Check sheet for the modelled part. Datum: model origin and axes. Units: mm. Round coordinates to 2 decimals unless told otherwise and drop trailing zeros. Order: outer loops, then holes, each group sorted by start corner. A loop starts at its lowest first (then second) coordinate and runs counter-clockwise, first axis right, second up. Notation, with made-up numbers: (28.25, 29) -> (74.25, 29) arc R17 cw to (74.25, 61) -> close; hole circle Ø3 at (-34, 3.25). An arc over 180 degrees is marked (long way). Use CSV: the item, a comma, the result in double quotes.
```python
from build123d import *

# Parameters (mm, degrees)
SKETCH1_R           = 9.5
SKETCH1_R_2         = 2
SKETCH1_R_3         = 2.5
BOSS_EXTRUDE1_DEPTH = 1.5


with BuildPart() as part:
    # Sketch1 → Boss-Extrude1 (new, symmetric)
    with BuildSketch(Plane.XY):
        with BuildLine():
            Line((165.5, 0), (165.5, 25))
            Line((165.5, 25), (84.5, 25))
            ThreePointArc((84.5, 25), (79.903805922, 26.903805922), (78, 31.5))
            Line((78, 31.5), (78, 72.5))
            ThreePointArc((78, 72.5), (77.267766953, 74.267766953), (75.5, 75))
            Line((75.5, 75), (-75.5, 75))
            ThreePointArc((-75.5, 75), (-77.267766953, 74.267766953), (-78, 72.5))
            Line((-78, 72.5), (-78, 31.5))
            ThreePointArc((-78, 31.5), (-79.903805922, 26.903805922), (-84.5, 25))
            Line((-84.5, 25), (-165.5, 25))
            Line((-165.5, 25), (-165.5, 0))
            Line((-165.5, 0), (165.5, 0))
        make_face()
        with Locations((0, 50)):
            Circle(SKETCH1_R, mode=Mode.SUBTRACT)
        with Locations((-65, 69)):
            Circle(SKETCH1_R_2, mode=Mode.SUBTRACT)
        with Locations((-39, 69)):
            Circle(SKETCH1_R_2, mode=Mode.SUBTRACT)
        with Locations((-13, 69)):
            Circle(SKETCH1_R_2, mode=Mode.SUBTRACT)
        with Locations((13, 69)):
            Circle(SKETCH1_R_2, mode=Mode.SUBTRACT)
        with Locations((39, 69)):
            Circle(SKETCH1_R_2, mode=Mode.SUBTRACT)
        with Locations((65, 69)):
            Circle(SKETCH1_R_2, mode=Mode.SUBTRACT)
        with Locations((-78, 12.5)):
            Circle(SKETCH1_R_3, mode=Mode.SUBTRACT)
        with Locations((78, 12.5)):
            Circle(SKETCH1_R_3, mode=Mode.SUBTRACT)
        with BuildLine():
            Line((-55, 60), (-25, 60))
            ThreePointArc((-25, 60), (-21.464466094, 58.535533906), (-20, 55))
            Line((-20, 55), (-20, 15))
            ThreePointArc((-20, 15), (-21.464466094, 11.464466094), (-25, 10))
            Line((-25, 10), (-55, 10))
            ThreePointArc((-55, 10), (-58.535533906, 11.464466094), (-60, 15))
            Line((-60, 15), (-60, 55))
            ThreePointArc((-60, 55), (-58.535533906, 58.535533906), (-55, 60))
        make_face(mode=Mode.SUBTRACT)
        with BuildLine():
            Line((-133, 17.5), (-95, 17.5))
            ThreePointArc((-95, 17.5), (-90, 12.5), (-95, 7.5))
            Line((-95, 7.5), (-133, 7.5))
            ThreePointArc((-133, 7.5), (-138, 12.5), (-133, 17.5))
        make_face(mode=Mode.SUBTRACT)
        with BuildLine():
            Line((133, 17.5), (95, 17.5))
            ThreePointArc((95, 17.5), (90, 12.5), (95, 7.5))
            Line((95, 7.5), (133, 7.5))
            ThreePointArc((133, 7.5), (138, 12.5), (133, 17.5))
        make_face(mode=Mode.SUBTRACT)
        with BuildLine():
            Line((55, 10), (25, 10))
            ThreePointArc((25, 10), (21.464466094, 11.464466094), (20, 15))
            Line((20, 15), (20, 55))
            ThreePointArc((20, 55), (21.464466094, 58.535533906), (25, 60))
            Line((25, 60), (55, 60))
            ThreePointArc((55, 60), (58.535533906, 58.535533906), (60, 55))
            Line((60, 55), (60, 15))
            ThreePointArc((60, 15), (58.535533906, 11.464466094), (55, 10))
        make_face(mode=Mode.SUBTRACT)
    extrude(amount=BOSS_EXTRUDE1_DEPTH, both=True)


solid = part.part
```
Q1. Go/stop test with flat-tipped pins: pin 1 (3 mm diameter, centred on x = -65, y = 69, fed in from +Z); pin 2 (1 mm diameter, centred on x = 126, z = 0.5, fed in from -Y); pin 3 (1.5 mm diameter, centred on y = 32.5, z = 0, fed in from +X); pin 4 (0.9 mm diameter, centred on y = 54.5, z = -0.5, fed in from -X). Record where each tip stops, or that it passes through.
Result sheet:
pin 1,"passes through"
pin 2,"stops at y = 0"
pin 3,"stops at x = 78"
pin 4,"stops at x = -78"
Q2. Sectioned sample at A-A, the plane x = -115.5. Enter the section's corners in (y, z).
Result sheet:
outline,"(0, -1.5) -> (7.5, -1.5) -> (7.5, 1.5) -> (0, 1.5) -> close; (17.5, -1.5) -> (25, -1.5) -> (25, 1.5) -> (17.5, 1.5) -> close"
Q3. Sectioned sample at B-B, the plane x = 44.5. Enter the section's corners in (y, z), then the cut area to 3 significant figures.
Result sheet:
outline,"(0, -1.5) -> (10, -1.5) -> (10, 1.5) -> (0, 1.5) -> close; (60, -1.5) -> (75, -1.5) -> (75, 1.5) -> (60, 1.5) -> close"
area,"75.0 mm^2"
Q4. Mould release check, pull along X, two halves, no side actions. Record for faces 1 (the face through (-1.24, 59.42, -0.02)), 2 (the face through (-2, 30, -1.5)), 3 (the face through (-79.854, 26.955, 0.021)): pulls with the +X half, pulls with the -X half, needs draft (parallel to the pull), parting line crosses it, or undercut.
Result sheet:
face 1,"undercut"
face 2,"needs draft"
face 3,"pulls with the -X half"
Q5. Sectioned sample at C-C, the plane z = -0.8. State how many separate pieces and enclosed holes the cut face has, then the cut area to 3 significant figures.
Result sheet:
separate pieces,"1"
enclosed holes,"13"
area,"10,800 mm^2"
Q6. Scan lines: L1, parallel to Y at x = 39, z = 0.2; L2, parallel to X at y = 24.5, z = -0.3; L3, parallel to X at y = 38, z = -0.5. Record each from-to range of solid material in increasing order.
Result sheet:
L1,"y = 0 to 10, 60 to 67, 71 to 75"
L2,"x = -165.5 to -60, -20 to 20, 60 to 165.5"
L3,"x = -78 to -60, -20 to 20, 60 to 78"
